Work out the finished part from the listing and answer in its coordinate system (mm). Coordinates: 2 decimals unless noted, no trailing zeros. Loops run counter-clockwise (first coordinate to the right, second up) from the corner with the lowest first, then second, coordinate; pieces in that order, holes last. Notation, with made-up numbers: M 69.5,20.25 L 126.5,20.25 A9 ccw 126.5,35.25 Z; hole C -20,50 d8. An arc over 180 degrees is marked long. Write each question's results on one line, items separated by ' | '.
```python
from build123d import *

# Parameters (mm, degrees)
F0_W     = 42.3
F0_H     = 42.3
F0_W_2   = 31
F0_H_2   = 31
F0_R     = 11.25
F1_DEPTH = 12.5
F2_R     = 5
F3_R     = 5
F4_D     = 5


with BuildPart() as f1:
    # F0 (on Top) → F1 (new body)
    with BuildSketch(Plane.XY):
        Rectangle(F0_W, F0_H)
        Rectangle(F0_W_2, F0_H_2, mode=Mode.SUBTRACT)
        Rectangle(F0_W_2, F0_H_2)
        Circle(F0_R, mode=Mode.SUBTRACT)
    extrude(amount=-F1_DEPTH)

    # F2
    f2_edges = [f1.edges().sort_by_distance(p)[0] for p in [
        (21.15, -21.15, -6.25),
        (-21.15, 21.15, -6.25),
        (21.15, 21.15, -6.25),
    ]]
    fillet(f2_edges, radius=F2_R)

    # F3
    f3_edges = [f1.edges().sort_by_distance(p)[0] for p in [
        (-21.15, -21.15, -6.25),
    ]]
    fillet(f3_edges, radius=F3_R)

    # F4 (through all)
    with Locations(Plane.XY):
        with Locations((-15.5, -15.5), (-15.5, 15.5), (15.5, 15.5), (15.5, -15.5)):
            Hole(F4_D / 2)


solid = f1.part
```
1) Find section A-A, the plane x = 13.5. Give the vertices of the cut face in (y, z).
Check result:
outline: M -21.15,-12.5 L -17,-12.5 L -17,0 L -21.15,0 Z; M -14,-12.5 L 14,-12.5 L 14,0 L -14,0 Z; M 17,-12.5 L 21.15,-12.5 L 21.15,0 L 17,0 Z
2) Straight lines are drawn through the part: probe 1 along Y at (x, z) = (15.5, -9.5); probe 2 along Y at (x, z) = (0, -2.25); probe 3 along X at (y, z) = (-15, -5.25). For each, find the intervals that lie inside material, in ascending order. Write a range as [from, to].
Check result:
probe 1: [-21.15, -18], [-13, 13], [18, 21.15] | probe 2: [-21.15, -11.25], [11.25, 21.15] | probe 3: [-21.15, -17.95], [-13.05, 13.05], [17.95, 21.15]
3) For a pull along X with two mould halves and no side action, classify faces 1 (the face through (0, -21.15, -6)), 2 (the face through (5.19, -9.98, -6.16)), 3 (the face through (17.5, 14, -6.3)), 4 (the face through (-19.72, 19.65, -6.34)) as released by +X, released by -X, zero draft, split by the parting line, or undercut.
Check result:
face 1: zero draft | face 2: undercut | face 3: undercut | face 4: released by -X
4) Find section D-D, the plane y = 0. Give the vertices of the cut face in (x, z), and give its area (4 significant figures).
Check result:
outline: M -21.15,-12.5 L -11.25,-12.5 L -11.25,0 L -21.15,0 Z; M 11.25,-12.5 L 21.15,-12.5 L 21.15,0 L 11.25,0 Z | area: 247.5 mm^2
5) Find section C-C, the plane z = -11. Give the vertices of the cut face in (x, y).
Check result:
outline: M -21.15,-16.15 A5 ccw -16.15,-21.15 L 16.15,-21.15 A5 ccw 21.15,-16.15 L 21.15,16.15 A5 ccw 16.15,21.15 L -16.15,21.15 A5 ccw -21.15,16.15 Z; hole C -15.5,-15.5 d5; hole C -15.5,15.5 d5; hole C 0,0 d22.5; hole C 15.5,-15.5 d5; hole C 15.5,15.5 d5
6) Find section B-B, the plane y = -15.5. Give the vertices of the cut face in (x, z), and give its area (3 significant figures).
Check result:
outline: M -21.15,-12.5 L -18,-12.5 L -18,0 L -21.15,0 Z; M -13,-12.5 L 13,-12.5 L 13,0 L -13,0 Z; M 18,-12.5 L 21.15,-12.5 L 21.15,0 L 18,0 Z | area: 404 mm^2
